The model under review builds one solid part; all positions refer to its coordinate system, in mm. Face numbers are marked on the shaded views. A direction names the side the tool comes from. Round coordinates to 2 decimals unless told otherwise and drop trailing zeros. Write each loop counter-clockwise with the first axis right and the second up, starting at its lowest first coordinate (ties: lowest second). Pieces come first, ordered by that corner, then holes. Notation, with made-up numbers: M 20,17 L 72,17 A6 ccw 72,27 Z; hole C 42,18 d7. An arc over 180 degrees is marked long. One line per item, written item: value. Start each with the question number.
1) Tool access review of the marked faces 4, 5, 6, 7 and 8: name each direction out of +Z, -Z, +X, -X, +Y, -Y from which nothing blocks a thin tool from reaching the whole face with its end or side.
2) Take a section at C-C, the plane x = 6.5. Write out the cut boundary in (y, z), and give its area (3 significant figures).
3) Take a section at B-B, the plane y = 11.75. State how many separate pieces and enclosed holes the cut face has, and give its area (3 significant figures).
4) For P1, Ø2, axis at x = 19, z = -2.5, coming from the -Y side; P2, Ø2, axis at x = -52, y = 5, coming from the +Z side; P3, Ø7, axis at x = 23, y = 7.5, coming from the +Z side, all flat-tipped, find the tip position at first contact; note any pin that passes through.
5) Mouldability with a two-part tool opening along X and no side actions: class the marked faces 1, 2 and 3 as +X half, -X half, draft (parallel to the pull), parting line (faces both ways), or undercut.
6) Take a section at A-A, the plane z = 0. Write out the cut boundary in (x, y).
7) Wall thickness on probe 1 along X at (y, z) = (12.75, 3.5); probe 2 along X at (y, z) = (12, 1); probe 3 along X at (y, z) = (8.75, 6): over which ranges is each line inside the solid? List them lowest first.
8) Take a section at D-D, the plane x = 40.5. Write out the cut boundary in (y, z), and give its area (3 significant figures).
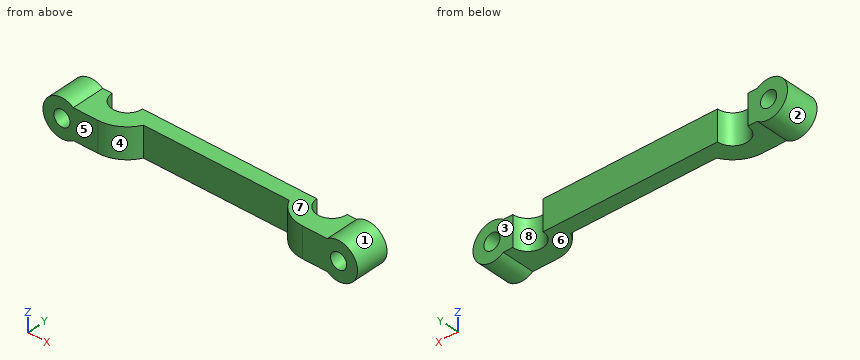
from build123d import *

# Parameters (mm, degrees)
BOSS_EXTRUDE1_DEPTH     = 13.89888
CUT_EXTRUDE1_DEPTH      = 69.830593656
CUT_EXTRUDE1_DEPTH_BACK = 69.830593656
CUT_EXTRUDE2_DEPTH      = 69.830593656
F_1_4_CLEARANCE_HOLE1_D = 6.7564


with BuildPart() as part:
    # Sketch1 → Boss-Extrude1 (new body)
    with BuildSketch(Plane(origin=(0, 0, 0), x_dir=(1, 0, 0), z_dir=(0, 1, 0))):
        with BuildLine():
            Line((-53.18125, 6.35), (53.18125, 6.35))
            ThreePointArc((53.18125, 6.35), (65.88125, 0), (53.18125, -6.35))
            Line((53.18125, -6.35), (-53.18125, -6.35))
            ThreePointArc((-53.18125, -6.35), (-65.88125, 0), (-53.18125, 6.35))
        make_face()
    extrude(amount=BOSS_EXTRUDE1_DEPTH)

    # Sketch2 → Cut-Extrude1 (cut, two sides: drawn at the far end of the back side and taken through both)
    with BuildSketch(Plane.XY.offset(6.35).offset(-CUT_EXTRUDE1_DEPTH_BACK)):
        with BuildLine():
            Line((-49.2125, 13.89888), (-36.5125, 13.89888))
            ThreePointArc((-36.5125, 13.89888), (-42.8625, 7.54888), (-49.2125, 13.89888))
        make_face()
        with BuildLine():
            Line((36.5125, 13.89888), (49.2125, 13.89888))
            ThreePointArc((49.2125, 13.89888), (42.8625, 7.54888), (36.5125, 13.89888))
        make_face()
    extrude(amount=CUT_EXTRUDE1_DEPTH + CUT_EXTRUDE1_DEPTH_BACK, mode=Mode.SUBTRACT)

    # Sketch3 → Cut-Extrude2 (cut, through all)
    with BuildSketch(Plane(origin=(0, 0, -6.35), x_dir=(-1, 0, 0), z_dir=(0, 0, -1))):
        with BuildLine():
            Line((30.498990577, 7.54888), (-30.498990577, 7.54888))
            ThreePointArc((-30.498990577, 7.54888), (-35.619538684, 2.036402323), (-42.8625, 0))
            Line((-42.8625, 0), (42.8625, 0))
            ThreePointArc((42.8625, 0), (35.619538684, 2.036402323), (30.498990577, 7.54888))
        make_face()
    extrude(amount=-CUT_EXTRUDE2_DEPTH, mode=Mode.SUBTRACT)

    # 1/4 Clearance Hole1 (through all)
    with Locations(Plane(origin=(0, 0, 0), x_dir=(-1, 0, 0), z_dir=(0, -1, 0))):
        with Locations((57.94375, 0), (-57.94375, 0)):
            Hole(F_1_4_CLEARANCE_HOLE1_D / 2)


solid = part.part
Checked values:
1. face 4: +Z, -Z, -Y
1. face 5: +Z, -Z, +X, -X, -Y
1. face 6: -Z, +Y, -Y
1. face 7: +Z, +Y, -Y
1. face 8: +Z, -Z, +Y
2. outline: M 7.55,-6.35 L 13.9,-6.35 L 13.9,6.35 L 7.55,6.35 Z
2. area: 80.6 mm2
3. separate pieces: 3
3. enclosed holes: 2
3. area: 1,320 mm2
4. P1: stops at y = 7.55
4. P2: stops at z = 6.35
4. P3: stops at z = 6.35
5. face 1: undercut
5. face 2: undercut
5. face 3: draft
6. outline: M -65.88,0 L -61.32,0 L -61.32,13.9 L -65.88,13.9 Z; M -54.57,0 L -42.86,0 A13.9 ccw -30.5,7.55 L 30.5,7.55 A13.9 ccw 42.86,0 L 54.57,0 L 54.57,13.9 L 49.21,13.9 A6.35 cw 36.51,13.9 L -36.51,13.9 A6.35 cw -49.21,13.9 L -54.57,13.9 Z; M 61.32,0 L 65.88,0 L 65.88,13.9 L 61.32,13.9 Z
7. probe 1: x = -65.07 to -49.11, -36.62 to 36.62, 49.11 to 65.07
7. probe 2: x = -65.82 to -61.17, -54.72 to -48.92, -36.8 to 36.8, 48.92 to 54.72, 61.17 to 65.82
7. probe 3: x = -63.14 to -46.58, -39.15 to 39.15, 46.58 to 63.14
8. outline: M 0.2,-6.35 L 8,-6.35 L 8,6.35 L 0.2,6.35 Z
8. area: 99.1 mm2
